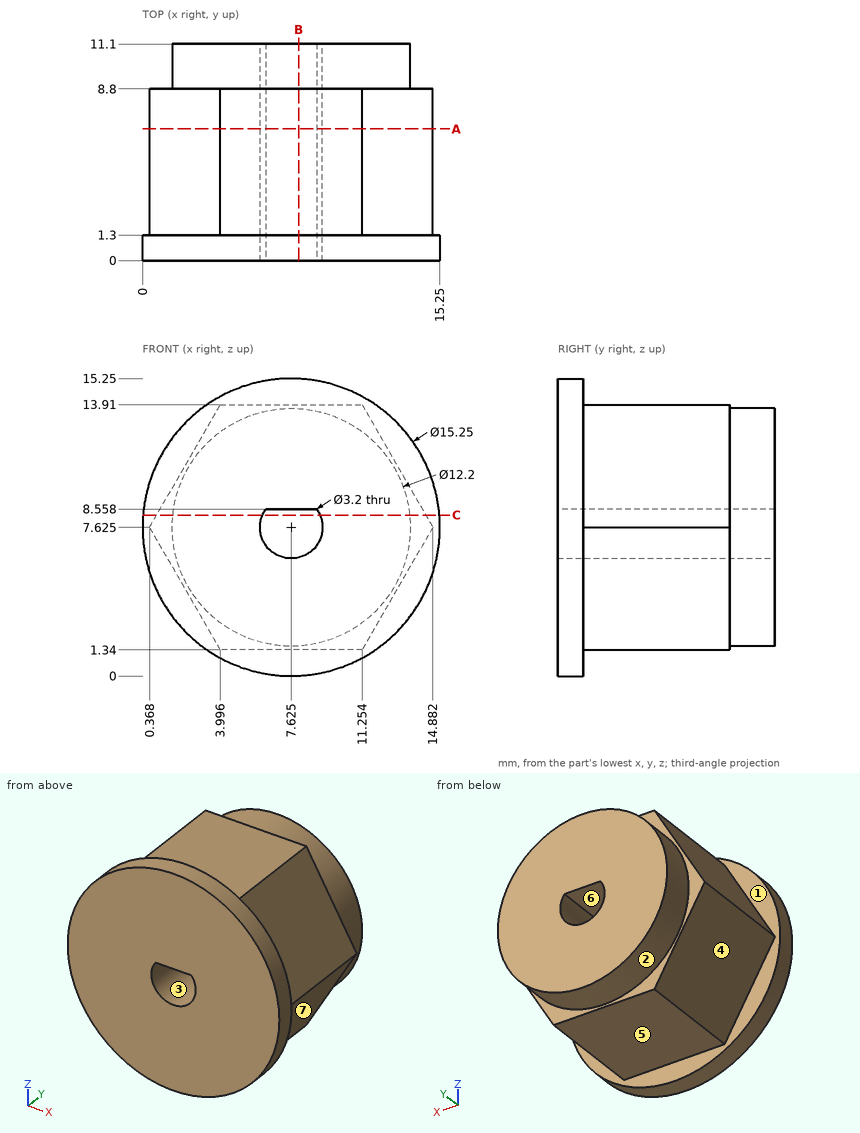
Answer from the drawing. Dimensions are ordinates in mm from the lowest x, y and z of the part. A direction names the side the tool comes from. Coordinates: 2 decimals unless noted, no trailing zeros. Loops run counter-clockwise (first coordinate to the right, second up) from the corner with the lowest first, then second, coordinate; pieces in that order, holes last. Notation, with made-up numbers: (-25.5, 71) -> (-3.5, 71) arc R22 cw to (-3.5, 92) -> close; hole circle Ø5 at (-33.5, 35.25). An arc over 180 degrees is marked (long way). Answer in a Markdown table with one row per item.
Item 1: For the marked faces 5, 6 and 7, determine the directions among +Z, -Z, +X, -X, +Y, -Y from which every point of the face is accessible in a straight line to the end or side of a thin tool.
Returned:
| item | result |
|---|---|
| face 5 | -Z, +X, -X, +Y |
| face 6 | +Y, -Y |
| face 7 | -Z, +X, +Y |
Item 2: Straight lines are drawn through the part: line 1 along Z through (x, y) = (7, 1.5); line 2 along Y through (x, z) = (1.5, 10); line 3 along Y through (x, z) = (9, 1.5). For each, find the intervals that lie inside material, in ascending order. Write a range as [from, to].
Returned:
| item | result |
|---|---|
| line 1 | z = [1.34, 6.15], [8.56, 13.91] |
| line 2 | y = [0, 1.3] |
| line 3 | y = [0, 8.8] |
Item 3: For a pull along Z with two mould halves and no side action, classify the marked faces 1, 2, 3 and 4 as released by +Z, released by -Z, zero draft, split by the parting line, or undercut.
Returned:
| item | result |
|---|---|
| face 1 | zero draft |
| face 2 | split by the parting line |
| face 3 | undercut |
| face 4 | released by -Z |
Item 4: A cutting plane is placed at B-B on x = 8. Determine the outline of the cut face in (y, z).
Returned:
| item | result |
|---|---|
| outline | (0, 0.01) -> (1.3, 0.01) -> (1.3, 1.34) -> (8.8, 1.34) -> (8.8, 1.54) -> (11.1, 1.54) -> (11.1, 6.07) -> (0, 6.07) -> close; (0, 8.56) -> (11.1, 8.56) -> (11.1, 13.71) -> (8.8, 13.71) -> (8.8, 13.91) -> (1.3, 13.91) -> (1.3, 15.24) -> (0, 15.24) -> close |
Item 5: A cutting plane is placed at C-C on z = 8.25. Determine the outline of the cut face in (x, y) (1 decimal).
Returned:
| item | result |
|---|---|
| outline | (0, 0) -> (6.2, 0) -> (6.2, 11.1) -> (1.6, 11.1) -> (1.6, 8.8) -> (0.7, 8.8) -> (0.7, 1.3) -> (0, 1.3) -> close; (9.1, 0) -> (15.2, 0) -> (15.2, 1.3) -> (14.5, 1.3) -> (14.5, 8.8) -> (13.7, 8.8) -> (13.7, 11.1) -> (9.1, 11.1) -> close |
Item 6: Each of these flat-tipped pins is pushed along its axis until it touches: P1, Ø3, axis at x = 7.5, y = 4.5, coming from the -Z side; P2, Ø2, axis at y = 1.5, z = 2.5, coming from the +X side (1 decimal); P3, Ø2, axis at x = 8, y = 4.5, coming from the +Z side. Where does it stop, or does it pass through?
Returned:
| item | result |
|---|---|
| P1 | stops at z = 1.34 |
| P2 | stops at x = 14 |
| P3 | stops at z = 13.91 |
Item 7: A cutting plane is placed at A-A on y = 6.75. Determine the outline of the cut face in (x, z) (1 decimal), plus the area to 3 significant figures.
Returned:
| item | result |
|---|---|
| outline | (0.4, 7.6) -> (4, 1.3) -> (11.3, 1.3) -> (14.9, 7.6) -> (11.3, 13.9) -> (4, 13.9) -> close; hole (6.3, 8.6) arc R1.6 ccw (long way) to (8.9, 8.6) -> close |
| area | 130 mm^2 |
